```python
from build123d import *

# Parameters (mm, degrees)
REVOLUTION_ANGLE = 270


with BuildPart() as part:
    # Sketch → Revolution (revolve)
    with BuildSketch(Plane.XY):
        Polygon((0, -22.5), (-75, -22.5), (-75, -32.5), (-55, -32.5), (-55, -57.5), (-88, -57.5), (-88, -80), (-105, -80), (-105, -100), (-70, -100), (-70, -77.5), (-35, -77.5), (-35, -55), (0, -55), align=None)
    revolve(axis=Axis((0, 0, 0), (1, 0, 0)), revolution_arc=REVOLUTION_ANGLE)


solid = part.part
```
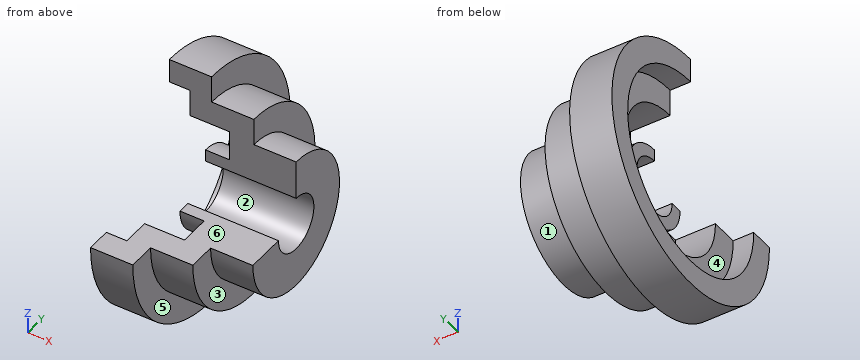
Verification items for the finished model (mm, model axes). Face numbers are marked on the shaded views. A direction names the side the tool comes from. Give positions to 0.01 mm unless a question says otherwise; leave off trailing zeros. Loops run counter-clockwise (first coordinate to the right, second up) from the corner with the lowest first, then second, coordinate; pieces in that order, holes last. Notation, with made-up numbers: M 60.5,1 L 83.5,1 A25 ccw 83.5,36 Z; hole C 19,15 d6. An arc over 180 degrees is marked long. One line per question, with ' | ' between items.
Item 1: Depth check by flat-ended pin: P1, Ø6, axis at x = -80.5, y = 72.5, coming from the +Z side; P2, Ø12, axis at x = -51, y = 67.5, coming from the +Z side; P3, Ø5, axis at x = -55, y = -74, coming from the -Z side. Enter the tip coordinate at first touch or a pass-through.
Completed:
P1: stops at z = 71.9 | P2: stops at z = 47.16 | P3: stops at z = -29.9
Item 2: Section check A-A, the plane z = -44. Record the cut outline in (x, y).
Completed:
outline: M -105,-89.8 L -70,-89.8 L -70,-63.8 L -35,-63.8 L -35,-33 L 0,-33 L 0,33 L -35,33 L -35,63.8 L -70,63.8 L -70,89.8 L -105,89.8 L -105,66.81 L -88,66.81 L -88,37.02 L -55,37.02 L -55,-37.02 L -88,-37.02 L -88,-66.81 L -105,-66.81 Z
Item 3: Tool access check on the marked faces 4, 5 and 6. Record the directions out of +Z, -Z, +X, -X, +Y, -Y that give a thin tool (end or side, any length) a straight path to the whole face; none if there is none.
Completed:
face 4: -X | face 5: +X | face 6: +Z, +X, -X, -Y
Item 4: Section check D-D, the plane y = 42.5. Record the cut outline in (x, z).
Completed:
outline: M -105,-90.52 L -70,-90.52 L -70,-64.81 L -35,-64.81 L -35,-34.91 L 0,-34.91 L 0,34.91 L -35,34.91 L -35,64.81 L -70,64.81 L -70,90.52 L -105,90.52 L -105,67.78 L -88,67.78 L -88,38.73 L -55,38.73 L -55,-38.73 L -88,-38.73 L -88,-67.78 L -105,-67.78 Z
Item 5: Draft check along Y on the marked faces 1, 2 and 3. Enter one of: +Y half, -Y half, draft (parallel to the pull), parting line (faces both ways), or undercut.
Completed:
face 1: parting line | face 2: undercut | face 3: draft
Item 6: Section check C-C, the plane y = -62.5. Record the cut outline in (x, z), plus the area to 3 significant figures.
Completed:
outline: M -105,-78.06 L -70,-78.06 L -70,-45.83 L -35,-45.83 L -35,0 L -88,0 L -88,-49.94 L -105,-49.94 Z | area: 3,490 mm^2
Item 7: Section check B-B, the plane x = -24.5. Record the cut outline in (y, z), plus the area to 3 significant figures.
Completed:
outline: M -55,0 A55 ccw long 0,55 L 0,22.5 A22.5 cw long -22.5,0 Z | area: 5,930 mm^2
Item 8: Thickness scan on line 1 (X direction, y = 39, z = -77); line 2 (X direction, y = 49, z = -10); line 3 (Z direction, x = -67.5, y = -5.5). Record the ranges inside material, lowest first. Write a range as [from, to].
Completed:
line 1: x = [-105, -70] | line 2: x = [-55, 0] | line 3: z = [-77.3, -57.24], [-32.03, -21.82]
